```python
from build123d import *

# Parameters (mm, degrees)
MODEL_R                 = 14.5
SALIENTE_EXTRUIR1_DEPTH = 3


with BuildPart() as part:
    # Model → Saliente-Extruir1 (new body)
    with BuildSketch(Plane.XY):
        with BuildLine():
            Line((47.37313945, 289.774034505), (50.166269539, 294.611877731))
            ThreePointArc((50.166269539, 294.611877731), (44.006853837, 296.990237588), (37.483463439, 298.010225383))
            Line((37.483463439, 298.010225383), (37.483463439, 292.423965206))
            Line((37.483463439, 292.423965206), (34.483463439, 292.423965206))
            Line((34.483463439, 292.423965206), (34.483463439, 298.010225383))
            ThreePointArc((34.483463439, 298.010225383), (27.960073041, 296.990237588), (21.800657339, 294.611877731))
            Line((21.800657339, 294.611877731), (24.593787428, 289.774034505))
            Line((24.593787428, 289.774034505), (21.995711217, 288.274034505))
            Line((21.995711217, 288.274034505), (19.202581128, 293.111877731))
            ThreePointArc((19.202581128, 293.111877731), (14.063153222, 288.966847189), (9.91812268, 283.827419284))
            Line((9.91812268, 283.827419284), (14.755965907, 281.034289195))
            Line((14.755965907, 281.034289195), (13.255965907, 278.436212983))
            Line((13.255965907, 278.436212983), (8.41812268, 281.229343072))
            ThreePointArc((8.41812268, 281.229343072), (6.039762824, 275.069927371), (5.019775028, 268.546536973))
            Line((5.019775028, 268.546536973), (10.606035206, 268.546536973))
            Line((10.606035206, 268.546536973), (10.606035206, 265.546536973))
            Line((10.606035206, 265.546536973), (5.019775028, 265.546536973))
            ThreePointArc((5.019775028, 265.546536973), (6.039762824, 259.023146574), (8.41812268, 252.863730873))
            Line((8.41812268, 252.863730873), (13.255965907, 255.656860962))
            Line((13.255965907, 255.656860962), (14.755965907, 253.05878475))
            Line((14.755965907, 253.05878475), (9.91812268, 250.265654662))
            ThreePointArc((9.91812268, 250.265654662), (14.063153222, 245.126226756), (19.202581128, 240.981196214))
            Line((19.202581128, 240.981196214), (21.995711217, 245.81903944))
            Line((21.995711217, 245.81903944), (24.593787428, 244.31903944))
            Line((24.593787428, 244.31903944), (21.800657339, 239.481196214))
            ThreePointArc((21.800657339, 239.481196214), (27.960073041, 237.102836358), (34.483463439, 236.082848562))
            Line((34.483463439, 236.082848562), (34.483463439, 241.66910874))
            Line((34.483463439, 241.66910874), (37.483463439, 241.66910874))
            Line((37.483463439, 241.66910874), (37.483463439, 236.082848562))
            ThreePointArc((37.483463439, 236.082848562), (44.006853837, 237.102836358), (50.166269539, 239.481196214))
            Line((50.166269539, 239.481196214), (47.37313945, 244.31903944))
            Line((47.37313945, 244.31903944), (49.971215661, 245.81903944))
            Line((49.971215661, 245.81903944), (52.76434575, 240.981196214))
            ThreePointArc((52.76434575, 240.981196214), (57.903773656, 245.126226756), (62.048804198, 250.265654662))
            Line((62.048804198, 250.265654662), (57.210960972, 253.05878475))
            Line((57.210960972, 253.05878475), (58.710960972, 255.656860962))
            Line((58.710960972, 255.656860962), (63.548804198, 252.863730873))
            ThreePointArc((63.548804198, 252.863730873), (65.927164054, 259.023146574), (66.94715185, 265.546536973))
            Line((66.94715185, 265.546536973), (61.360891672, 265.546536973))
            Line((61.360891672, 265.546536973), (61.360891672, 268.546536973))
            Line((61.360891672, 268.546536973), (66.94715185, 268.546536973))
            ThreePointArc((66.94715185, 268.546536973), (65.927164054, 275.069927371), (63.548804198, 281.229343072))
            Line((63.548804198, 281.229343072), (58.710960972, 278.436212983))
            Line((58.710960972, 278.436212983), (57.210960972, 281.034289195))
            Line((57.210960972, 281.034289195), (62.048804198, 283.827419284))
            ThreePointArc((62.048804198, 283.827419284), (57.903773656, 288.966847189), (52.76434575, 293.111877731))
            Line((52.76434575, 293.111877731), (49.971215661, 288.274034505))
            Line((49.971215661, 288.274034505), (47.37313945, 289.774034505))
        make_face()
        with Locations((35.983463439, 267.046536973)):
            Circle(MODEL_R, mode=Mode.SUBTRACT)
    extrude(amount=SALIENTE_EXTRUIR1_DEPTH)


solid = part.part
```
Source: CAD feature listing. Evaluate the final solid. Frame: model axes, mm. A direction names the side the tool comes from. Give positions to 0.01 mm unless a question says otherwise; leave off trailing zeros. Write each loop counter-clockwise with the first axis right and the second up, starting at its lowest first coordinate (ties: lowest second). Pieces come first, ordered by that corner, then holes.
1. Section query A-A (x = 26.5). Return the cut outline in (y, z).
2. Section query D-D (x = 51.5). Return the cut outline in (y, z).
3. Section query B-B (x = 38.5). Return the cut outline in (y, z).
4. Section query C-C (y = 283). Return the cut outline in (x, z).
5. Pull-direction query (X, two-part tool) for faces 1 (the face through (10.871, 279.813, 1.479)), 2 (the face through (14.016, 279.753, 1.479)), 3 (the face through (44.096, 296.966, 1.479)), 4 (the face through (14, 245.19, 1.48)); classes: +X half, -X half, draft (parallel to the pull), parting line (faces both ways), or undercut.
6. First-contact query: pin 1 (1.5 mm diameter, centred on y = 267, z = 1, fed in from -X); pin 2 (1.5 mm diameter, centred on x = 65.5, z = 1.5, fed in from -Y); pin 3 (0.9 mm diameter, centred on x = 8, z = 1.5, fed in from -Y). Flat tips, straight axial feed; report the tip coordinate or a pass-through.
7. Access query for faces 5 (the face through (57.95, 254.34, 1.48)), 6 (the face through (6.064, 275.159, 1.479)). Directions: +Z, -Z, +X, -X, +Y, -Y. A direction counts if a zero-diameter tool reaches every point of the face in a straight line with its end or side. Return the directions, or none.
8. Material intervals for line 1 along Y through (x, z) = (61, 1.85); line 2 along Y through (x, z) = (58.5, 1.45); line 3 along X through (y, z) = (291.5, 0.55), sorted ascending.
Output values:
1. outline: (237.53, 0) - (256.08, 0) - (256.08, 3) - (237.53, 3) - close; (278.02, 0) - (296.56, 0) - (296.56, 3) - (278.02, 3) - close
2. outline: (243.17, 0) - (290.92, 0) - (290.92, 3) - (243.17, 3) - close
3. outline: (236.15, 0) - (252.77, 0) - (252.77, 3) - (236.15, 3) - close; (281.33, 0) - (297.94, 0) - (297.94, 3) - (281.33, 3) - close
4. outline: (11.35, 0) - (60.62, 0) - (60.62, 3) - (11.35, 3) - close
5. face 1: undercut
5. face 2: undercut
5. face 3: +X half
5. face 4: -X half
6. pin 1: stops at x = 10.61
6. pin 2: stops at y = 255.49
6. pin 3: stops at y = 252.86
7. face 5: +Z, -Z
7. face 6: +Z, -Z, -X, +Y
8. line 1: y = 248.74 to 250.87, 254.34 to 279.76, 283.22 to 285.35
8. line 2: y = 245.74 to 252.31, 255.29 to 278.8, 281.78 to 288.35
8. line 3: x = 16.93 to 20.13, 23.6 to 48.37, 51.83 to 55.04
